CAD build for the part. Positions are in the model's coordinates, mm. A direction names the side the tool comes from. Round coordinates to 2 decimals unless told otherwise and drop trailing zeros. Write each loop counter-clockwise with the first axis right and the second up, starting at its lowest first coordinate (ties: lowest second). Pieces come first, ordered by that corner, then holes. Notation, with made-up numbers: (71, 47) - (90, 47) arc R25 ccw to (90, 67) - close; hole circle Ø1 at (-17, -12.75). An arc over 180 degrees is marked (long way). Answer in a Markdown table with one row per item.
```python
from build123d import *

# Parameters (mm, degrees)
SKETCH_1_R          = 6
EXTRUDE_1_DEPTH     = 30
CUT_EXTRUDE_START   = -4
SKETCH_2_R          = 6
SKETCH_2_R_2        = 5
CUT_EXTRUDE_1_DEPTH = 4
SKETCH_3_R          = 1.25
CUT_EXTRUDE_2_DEPTH = 10


with BuildPart() as part:
    # ｽｹｯﾁ1 → ﾎﾞｽ - 押し出し1 (new body)
    with BuildSketch(Plane.XY):
        Circle(SKETCH_1_R)
    extrude(amount=EXTRUDE_1_DEPTH)

    # ｽｹｯﾁ2 → ｶｯﾄ - 押し出し1 (cut)
    with BuildSketch(Plane.XY.offset(30).offset(CUT_EXTRUDE_START)):
        Circle(SKETCH_2_R)
        Circle(SKETCH_2_R_2, mode=Mode.SUBTRACT)
    extrude(amount=CUT_EXTRUDE_1_DEPTH, mode=Mode.SUBTRACT)

    # ｽｹｯﾁ3 → ｶｯﾄ - 押し出し2 (cut)
    with BuildSketch(Plane.XY.offset(30)):
        Circle(SKETCH_3_R)
    extrude(amount=-CUT_EXTRUDE_2_DEPTH, mode=Mode.SUBTRACT)


solid = part.part
```
Q1. Drill centre lines: line 1 (Y direction, x = 0, z = 24); line 2 (X direction, y = 1, z = 24); line 3 (Y direction, x = 1.5, z = 10.5). Where is each one in solid material? Low to high.
Computed:
| item | result |
|---|---|
| line 1 | y = -6 to -1.25, 1.25 to 6 |
| line 2 | x = -5.92 to -0.75, 0.75 to 5.92 |
| line 3 | y = -5.81 to 5.81 |
Q2. Saw through at A-A on x = 0. List the corners of the cut face in (y, z).
Computed:
| item | result |
|---|---|
| outline | (-6, 0) - (6, 0) - (6, 26) - (5, 26) - (5, 30) - (1.25, 30) - (1.25, 20) - (-1.25, 20) - (-1.25, 30) - (-5, 30) - (-5, 26) - (-6, 26) - close |
Q3. Saw through at C-C on y = 3. List the corners of the cut face in (x, z).
Computed:
| item | result |
|---|---|
| outline | (-5.2, 0) - (5.2, 0) - (5.2, 26) - (4, 26) - (4, 30) - (-4, 30) - (-4, 26) - (-5.2, 26) - close |
Q4. Flat gauge pins, fed straight in: pin 1 (3 mm diameter, centred on x = -1.5, y = 0, fed in from -Z); pin 2 (0.8 mm diameter, centred on x = 0.5, y = -0.5, fed in from +Z); pin 3 (2 mm diameter, centred on y = 4.5, z = 26.5, fed in from -X); pin 4 (1.5 mm diameter, centred on x = -3.5, z = 3.5, fed in from +Y). Where does each tip first touch, or does it go through?
Computed:
| item | result |
|---|---|
| pin 1 | stops at z = 0 |
| pin 2 | stops at z = 20 |
| pin 3 | stops at x = -4.77 |
| pin 4 | stops at y = 5.33 |
Q5. 3-axis set-ups, long thin cutter, end or side, ignore diameter. For faces 1 (the flat face through (0, 0, 20)), 2 (the flat face through (1, -1, 30)): which of +Z, -Z, +X, -X, +Y, -Y reach the whole face in a straight line?
Computed:
| item | result |
|---|---|
| face 1 | +Z |
| face 2 | +Z, +X, -X, +Y, -Y |
Q6. Saw through at B-B on z = 27.5. List the corners of the cut face in (x, y).
Computed:
| item | result |
|---|---|
| outline | circle Ø10 at (0, 0); hole circle Ø2.5 at (0, 0) |
Q7. Saw through at D-D on z = 10.25. List the corners of the cut face in (x, y), then the cut area to 3 significant figures.
Computed:
| item | result |
|---|---|
| outline | circle Ø12 at (0, 0) |
| area | 113 mm2 |
Q8. Pull direction Y, two halves, no side cores. Call faces 3 (the cylindrical face through (-0.27, -1.22, 25.07)), 4 (the flat face through (0, 0, 0)), 5 (the cylindrical face through (-1.08, -4.88, 27.97)): released by +Y, released by -Y, zero draft, split by the parting line, or undercut.
Computed:
| item | result |
|---|---|
| face 3 | undercut |
| face 4 | zero draft |
| face 5 | split by the parting line |
